The listing builds one solid part. Answer for the finished solid, in the listing's coordinates (mm). A direction names the side the tool comes from. Round coordinates to 2 decimals unless told otherwise and drop trailing zeros. Order: outer loops, then holes, each group sorted by start corner. A loop starts at its lowest first (then second) coordinate and runs counter-clockwise, first axis right, second up. Notation, with made-up numbers: (21, 60.5) - (56, 60.5) arc R20 cw to (56, 64.5) - close; hole circle Ø11 at (73, 83.25). An arc over 180 degrees is marked (long way). Write item = value, one per line.
from build123d import *

# Parameters (mm, degrees)
SKETCH_1_R               = 32.5
EXTRUDE_1_DEPTH          = 35
SKETCH_2_R               = 52.5
EXTRUDE_2_DEPTH          = 12
EXTRUDE_3_DEPTH          = 35
CUT_EXTRUDE_2_DEPTH      = 21
SKETCH_7_R               = 8
SKETCH_7_R_2             = 13
CUT_EXTRUDE_3_DEPTH      = 88.5
SKETCH_8_R               = 4.5
CUT_EXTRUDE_4_DEPTH      = 48
PATTERN_CIRCULAR_1_COUNT = 4
SKETCH_9_R               = 20
CUT_EXTRUDE_5_DEPTH      = 21
SKETCH_10_R              = 26
CUT_EXTRUDE_6_DEPTH      = 27


with BuildPart() as part:
    # 草图1 → 凸台-拉伸1 (new body)
    with BuildSketch(Plane.XY):
        Circle(SKETCH_1_R)
    extrude(amount=-EXTRUDE_1_DEPTH)

    # 草图2 → 凸台-拉伸2 (add)
    with BuildSketch(Plane(origin=(0, 0, -35), x_dir=(-1, 0, 0), z_dir=(0, 0, -1))):
        Circle(SKETCH_2_R)
    extrude(amount=EXTRUDE_2_DEPTH)

    # 草图4 → 凸台-拉伸3 (add, symmetric)
    with BuildSketch(Plane(origin=(0, 0, 0), x_dir=(0, 0, -1), z_dir=(1, 0, 0))):
        with BuildLine():
            Line((51, 52.5), (107, 52.5))
            ThreePointArc((107, 52.5), (120.522961568, 42.123466631), (114, 26.375644347))
            Line((114, 26.375644347), (93, 14.251288694))
            Line((93, 14.251288694), (93, -14.251288694))
            Line((93, -14.251288694), (114, -26.375644347))
            ThreePointArc((114, -26.375644347), (120.522961568, -42.123466631), (107, -52.5))
            Line((107, -52.5), (51, -52.5))
            ThreePointArc((51, -52.5), (48.171572875, -51.328427125), (47, -48.5))
            Line((47, -48.5), (47, 48.5))
            ThreePointArc((47, 48.5), (48.171572875, 51.328427125), (51, 52.5))
        make_face()
    extrude(amount=EXTRUDE_3_DEPTH, both=True)

    # 草图6 → 切除-拉伸2 (cut, symmetric)
    with BuildSketch(Plane(origin=(0, 0, 0), x_dir=(0, 0, -1), z_dir=(1, 0, 0))):
        with BuildLine():
            Line((107, 52.5), (51, 52.5))
            ThreePointArc((51, 52.5), (48.171572875, 51.328427125), (47, 48.5))
            Line((47, 48.5), (47, 39.131189606))
            Line((47, 39.131189606), (47, -39.131189606))
            Line((47, -39.131189606), (47, -48.5))
            ThreePointArc((47, -48.5), (48.171572875, -51.328427125), (51, -52.5))
            Line((51, -52.5), (107, -52.5))
            ThreePointArc((107, -52.5), (120.522961568, -42.123466631), (114, -26.375644347))
            Line((114, -26.375644347), (93, -14.251288694))
            Line((93, -14.251288694), (93, 14.251288694))
            Line((93, 14.251288694), (114, 26.375644347))
            ThreePointArc((114, 26.375644347), (120.522961568, 42.123466631), (107, 52.5))
        make_face()
    extrude(amount=CUT_EXTRUDE_2_DEPTH, both=True, mode=Mode.SUBTRACT)

    # 草图7 → 切除-拉伸3 (cut, through all)
    with BuildSketch(Plane(origin=(35, 0, 0), x_dir=(0, 0, -1), z_dir=(1, 0, 0))):
        with Locations((107, 38.5)):
            Circle(SKETCH_7_R)
        with Locations((107, -38.5)):
            Circle(SKETCH_7_R)
        with Locations((67, 0)):
            Circle(SKETCH_7_R_2)
    extrude(amount=-CUT_EXTRUDE_3_DEPTH, mode=Mode.SUBTRACT)

    # 草图8 → 切除-拉伸4 (cut, through all)
    with BuildSketch(Plane(origin=(0, 0, -47), x_dir=(-1, 0, 0), z_dir=(0, 0, -1))):
        with Locations((0, 45)):
            Circle(SKETCH_8_R)
    cut_extrude_4 = extrude(amount=-CUT_EXTRUDE_4_DEPTH, mode=Mode.SUBTRACT)

    # 阵列(圆周)1: 切除-拉伸4 ×4 about axis
    pattern_circular_1_axis = Axis((0, 0, 0), (0, 0, 1))
    for i in range(1, PATTERN_CIRCULAR_1_COUNT):
        add(cut_extrude_4.rotate(pattern_circular_1_axis, i * 360 / PATTERN_CIRCULAR_1_COUNT), mode=Mode.SUBTRACT)

    # 草图9 → 切除-拉伸5 (cut)
    with BuildSketch(Plane(origin=(0, 0, -47), x_dir=(-1, 0, 0), z_dir=(0, 0, -1))):
        Circle(SKETCH_9_R)
    extrude(amount=-CUT_EXTRUDE_5_DEPTH, mode=Mode.SUBTRACT)

    # 草图10 → 切除-拉伸6 (cut, through all)
    with BuildSketch(Plane(origin=(0, 0, -26), x_dir=(-1, 0, 0), z_dir=(0, 0, -1))):
        Circle(SKETCH_10_R)
    extrude(amount=-CUT_EXTRUDE_6_DEPTH, mode=Mode.SUBTRACT)


solid = part.part
Q1. Find the intervals of material crossed by line 1 (X direction, y = -39, z = -98); line 2 (Y direction, x = -25, z = -67); line 3 (Y direction, x = 26, z = -107), in increasing order. Write a range as from..to.
Model answer:
line_1 = -35..-21, 21..35
line_2 = -52.5..-13, 13..52.5
line_3 = -52.5..-46.5, -30.5..-22.33, 22.33..30.5, 46.5..52.5
Q2. Section C-C on x = 45 is taken. Determine the outline of the cut face in (y, z), then the cut area to 3 significant figures.
Model answer:
outline = (-27.04, -47) - (-4.5, -47) - (-4.5, -35) - (-27.04, -35) - close; (4.5, -47) - (27.04, -47) - (27.04, -35) - (4.5, -35) - close
area = 541 mm^2
Q3. Section D-D on z = -44 is taken. Determine the outline of the cut face in (x, y), then the cut area to 3 significant figures.
Model answer:
outline = circle Ø105 at (0, 0); hole circle Ø9 at (-45, 0); hole circle Ø40 at (0, 0); hole circle Ø9 at (0, -45); hole circle Ø9 at (0, 45); hole circle Ø9 at (45, 0)
area = 7,150 mm^2
Q4. For faces 5 (the face through (35, 1, -85)), 6 (the face through (19, 12, -47)), 7 (the face through (-27.902, -20.229, -103.353)), 8 (the face through (-50.076, 15.77, -40.916)), determine the directions among +Z, -Z, +X, -X, +Y, -Y from which every point of the face is accessible in a straight line to the end or side of a thin tool.
Model answer:
face_5 = -Z, +X, +Y, -Y
face_6 = -Z, +Y, -Y
face_7 = -Z, +X, -X
face_8 = +Z
Q5. Section A-A on z = -67 is taken. Determine the outline of the cut face in (x, y).
Model answer:
outline = (-35, -52.5) - (-21, -52.5) - (-21, -13) - (-35, -13) - close; (-35, 13) - (-21, 13) - (-21, 52.5) - (-35, 52.5) - close; (21, -52.5) - (35, -52.5) - (35, -13) - (21, -13) - close; (21, 13) - (35, 13) - (35, 52.5) - (21, 52.5) - close
Q6. Section B-B on y = 8 is taken. Count the separate pieces of the cut face and the enclosed holes in it, then the cut area to 3 significant figures.
Model answer:
separate_pieces = 4
enclosed_holes = 0
area = 2,110 mm^2
Q7. Determine the mould class of faces 1 (the face through (28.1, 3.9, -79.4)), 2 (the face through (-27.902, -51.359, -48.203)), 3 (the face through (-27.9, 40.9, -114.63)), 4 (the face through (28.1, 20.4, -103.65)) for opening direction Z: released by +Z, released by -Z, zero draft, split by the parting line, or undercut.
Model answer:
face_1 = undercut
face_2 = released by +Z
face_3 = undercut
face_4 = released by -Z
Q8. Flat-ended cylindrical pins translate along their axes: P1, Ø10.5, axis at x = 0, y = -45, coming from the -Z side; P2, Ø10.5, axis at x = -45, y = 0, coming from the +Z side; P3, Ø2, axis at y = -12.5, z = -23, coming from the -X side. Find the tip coordinate at first contact, or state that the pin passes through.
Model answer:
P1 = -47
P2 = -35
P3 = -30.4
